from build123d import *

# Parameters (mm, degrees)
F1_DEPTH = 3


with BuildPart() as f1:
    # F0 (on Front) → F1 (new body)
    with BuildSketch(Plane.XZ):
        with BuildLine():
            Line((-20.945015, -5), (-11.508791, -5))
            ThreePointArc((-11.508791, -5), (7.107153, 1.562372), (14.154985, 20))
            Line((14.154985, 20), (4.154985, 20))
            Line((4.154985, 20), (4.154985, 17))
            Line((4.154985, 17), (-5.845015, 17))
            Line((-5.845015, 17), (-5.845015, 20))
            Line((-5.845015, 20), (-15.845015, 20))
            Line((-15.845015, 20), (-15.845015, 17))
            Line((-15.845015, 17), (-25.845015, 17))
            Line((-25.845015, 17), (-25.845015, 20))
            Line((-25.845015, 20), (-35.845015, 20))
            Line((-35.845015, 20), (-35.845015, 15))
            Line((-35.845015, 15), (-32.845015, 15))
            Line((-32.845015, 15), (-32.845015, 10))
            Line((-32.845015, 10), (-35.845015, 10))
            Line((-35.845015, 10), (-35.845015, 5))
            Line((-35.845015, 5), (-32.845015, 5))
            Line((-32.845015, 5), (-32.845015, 0))
            Line((-32.845015, 0), (-35.845015, 0))
            Line((-35.845015, 0), (-35.845015, -5))
            Line((-35.845015, -5), (-23.845015, -5))
            Line((-23.845015, -5), (-23.845015, 1))
            Line((-23.845015, 1), (-20.945015, 1))
            Line((-20.945015, 1), (-20.945015, -5))
        make_face()
    extrude(amount=F1_DEPTH)


solid = f1.part
Geometry check sheet. Reference: the model listing, model coordinates, mm. A direction names the side the tool comes from. Round coordinates to 2 decimals unless told otherwise and drop trailing zeros. Order: outer loops, then holes, each group sorted by start corner. A loop starts at its lowest first (then second) coordinate and runs counter-clockwise, first axis right, second up. Notation, with made-up numbers: M 34,75 L 53,75 A17 ccw 53,105 Z; hole C 42.25,63 d11. An arc over 180 degrees is marked long. Write each question's results on one line, items separated by ' | '. Start each with the question number.
1. Set-up check for faces 1 (the face through (-32.845, -1, 3)), 2 (the face through (-11, -1, 20)), 3 (the face through (-35.845, -1, -2)), 4 (the face through (-21, -1, 17)), 5 (the face through (-23.845, -1, -2)): record each of +Z, -Z, +X, -X, +Y, -Y from which the full face is reachable in a straight line by a thin tool's end or side.
2. Draft check along Z on faces 6 (the face through (-34, -1, 15)), 7 (the face through (-1, -1, 17)), 8 (the face through (-30, -1, -5)). Enter one of: pulls with the +Z half, pulls with the -Z half, needs draft (parallel to the pull), parting line crosses it, or undercut.
3. Go/stop test with flat-tipped pins: P1, Ø1.5, axis at y = -1, z = 2.5, coming from the -X side (3 decimals); P2, Ø0.9, axis at x = -22, y = -1, coming from the -Z side; P3, Ø1.5, axis at y = -1.5, z = -3.5, coming from the +X side. Record where each tip stops, or that it passes through.
4. Cross-section at B-B on z = -2.75. Record the boundary of the cut face in (x, y).
5. Cross-section at C-C on x = -19.5. Record the boundary of the cut face in (y, z), plus the area to 3 significant figures.
6. Material ranges on L1, parallel to Z at x = -27.5, y = -2.75; L2, parallel to Z at x = -19.5, y = -1.65; L3, parallel to X at y = -2.15, z = -2.25, recorded low to high. Write a range as from..to.
7. Cross-section at D-D on z = 10.5. Record the boundary of the cut face in (x, y).
8. Cross-section at A-A on y = -2.5. Record the boundary of the cut face in (x, z), plus the area to 3 significant figures.
Resolved:
1) face 1: -X, +Y, -Y | face 2: +Z, +X, -X, +Y, -Y | face 3: +Z, -Z, -X, +Y, -Y | face 4: +Z, +Y, -Y | face 5: -Z, +Y, -Y
2) face 6: undercut | face 7: pulls with the +Z half | face 8: pulls with the -Z half
3) P1: x = -32.845 | P2: z = 1 | P3: x = 0.96
4) outline: M -35.85,-3 L -23.85,-3 L -23.85,0 L -35.85,0 Z; M -20.95,-3 L 0.96,-3 L 0.96,0 L -20.95,0 Z
5) outline: M -3,-5 L 0,-5 L 0,17 L -3,17 Z | area: 66.0 mm2
6) L1: -5..20 | L2: -5..17 | L3: -35.85..-23.85, -20.95..1.93
7) outline: M -32.85,-3 L 12.84,-3 L 12.84,0 L -32.85,0 Z
8) outline: M -35.85,-5 L -23.85,-5 L -23.85,1 L -20.95,1 L -20.95,-5 L -11.51,-5 A23.5 ccw 14.15,20 L 4.15,20 L 4.15,17 L -5.85,17 L -5.85,20 L -15.85,20 L -15.85,17 L -25.85,17 L -25.85,20 L -35.85,20 L -35.85,15 L -32.85,15 L -32.85,10 L -35.85,10 L -35.85,5 L -32.85,5 L -32.85,0 L -35.85,0 Z | area: 1,030 mm2
